from build123d import *

# Parameters (mm, degrees)
SKETCH1_W           = 24
SKETCH1_H           = 24
SKETCH1_W_2         = 20
SKETCH1_H_2         = 20
BOSS_EXTRUDE1_DEPTH = 40
SKETCH2_R           = 5
BOSS_EXTRUDE2_DEPTH = 7


with BuildPart() as part:
    # Sketch1 → Boss-Extrude1 (new body)
    with BuildSketch(Plane(origin=(0, 0, 0), x_dir=(0, 0, -1), z_dir=(1, 0, 0))):
        Rectangle(SKETCH1_W, SKETCH1_H)
        Rectangle(SKETCH1_W_2, SKETCH1_H_2, mode=Mode.SUBTRACT)
    extrude(amount=BOSS_EXTRUDE1_DEPTH)

    # Sketch2 → Boss-Extrude2 (add)
    with BuildSketch(Plane(origin=(0, 0, -12), x_dir=(-1, 0, 0), z_dir=(0, 0, -1))):
        with Locations(Location((-20, 0, 0), (0, 0, 90))):
            Circle(SKETCH2_R)
    extrude(amount=BOSS_EXTRUDE2_DEPTH)


solid = part.part
The listing builds one solid part. Answer for the finished solid, in the listing's coordinates (mm). A direction names the side the tool comes from. Coordinates: 2 decimals unless noted, no trailing zeros. Loops run counter-clockwise (first coordinate to the right, second up) from the corner with the lowest first, then second, coordinate; pieces in that order, holes last. Notation, with made-up numbers: (-5.5, 36) -> (36.5, 36) arc R22 cw to (36.5, 62) -> close; hole circle Ø7 at (-16, 58). An arc over 180 degrees is marked (long way). Answer in a Markdown table with one row per item. Add a question column.
1. The part is cut by section C-C, the plane x = 11.5. Write down the section's boundary in (y, z), then the cut area to 3 significant figures.
2. The part is cut by section D-D, the plane y = 0. Write down the section's boundary in (x, z).
3. Flat-ended cylindrical pins translate along their axes: P1, Ø6, axis at x = 15, y = 1, coming from the -Z side; P2, Ø6, axis at x = 29, y = 1.5, coming from the -Z side. Find the tip coordinate at first contact, or state that the pin passes through.
4. The part is cut by section A-A, the plane y = 5.5. Write down the section's boundary in (x, z), then the cut area to 3 significant figures.
5. Determine the mould class of faces 4 (the flat face through (20, 12, 0)), 5 (the flat face through (20, 0, -10)), 6 (the flat face through (20, 0, 12)), 7 (the flat face through (20, 10, 0)) for opening direction Z: +Z half, -Z half, draft (parallel to the pull), parting line (faces both ways), or undercut.
6. Consider line 1 (Z direction, x = 16.5, y = -4.25); line 2 (Z direction, x = 18.5, y = -1.25). Determine where each line is inside the solid, lowest interval first. Write a range as [from, to].
7. For faces 1 (the flat face through (20, 0, -19)), 2 (the flat face through (15, -3, -12)), 3 (the flat face through (20, -10, 0)), determine the directions among +Z, -Z, +X, -X, +Y, -Y from which every point of the face is accessible in a straight line to the end or side of a thin tool.
Answer below:
| question | item | result |
|---|---|---|
| 1 | outline | (-12, -12) -> (12, -12) -> (12, 12) -> (-12, 12) -> close; hole (-10, -10) -> (10, -10) -> (10, 10) -> (-10, 10) -> close |
| 1 | area | 176 mm2 |
| 2 | outline | (0, -12) -> (15, -12) -> (15, -19) -> (25, -19) -> (25, -12) -> (40, -12) -> (40, -10) -> (0, -10) -> close; (0, 10) -> (40, 10) -> (40, 12) -> (0, 12) -> close |
| 3 | P1 | z = -19 |
| 3 | P2 | z = -12 |
| 4 | outline | (0, -12) -> (40, -12) -> (40, -10) -> (0, -10) -> close; (0, 10) -> (40, 10) -> (40, 12) -> (0, 12) -> close |
| 4 | area | 160 mm2 |
| 5 | face 4 | draft |
| 5 | face 5 | undercut |
| 5 | face 6 | +Z half |
| 5 | face 7 | undercut |
| 6 | line 1 | [-12, -10], [10, 12] |
| 6 | line 2 | [-19, -10], [10, 12] |
| 7 | face 1 | -Z, +X, -X, +Y, -Y |
| 7 | face 2 | -Z |
| 7 | face 3 | +X, -X |
